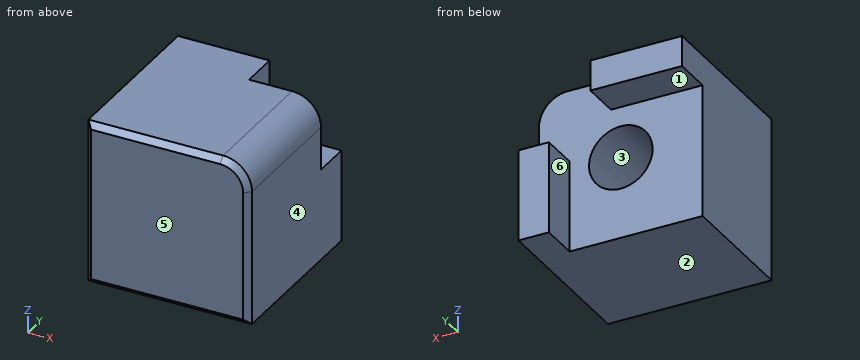
```python
from build123d import *

# Parameters (mm, degrees)
BASE_W                = 8.5
BASE_H                = 8.5
BOSS_EXTRUDE1_DEPTH   = 8.5
CUTOUT_W              = 7
CUTOUT_H              = 7
CUT_EXTRUDE1_DEPTH    = 1.5
SKETCH3_W             = 1.5
SKETCH3_H             = 1.5
CUT_EXTRUDE2_DEPTH    = 12.803071634
FILLET3_R             = 0.508
FILLET4_R             = 1.5
M4_TAPPED_HOLE1_D     = 3.3
M4_TAPPED_HOLE1_DEPTH = 5
M4_TAPPED_HOLE1_TIP   = 0.991420021
CUT_EXTRUDE3_START    = -1.5
CUT_EXTRUDE3_DEPTH    = 1.5
CHAMFER1_SIZE         = 0.3
SKETCH15_W            = 1.5875
SKETCH15_H            = 4.7625
SKETCH15_W_2          = 4.7625
SKETCH15_H_2          = 1.5875
BOSS_EXTRUDE2_DEPTH   = 2


with BuildPart() as part:
    # Base → Boss-Extrude1 (new body)
    with BuildSketch(Plane(origin=(0, 0, 0), x_dir=(1, 0, 0), z_dir=(0, 1, 0))):
        Rectangle(BASE_W, BASE_H)
    extrude(amount=-BOSS_EXTRUDE1_DEPTH)

    # Cutout → Cut-Extrude1 (cut)
    with BuildSketch(Plane(origin=(0, 0, 0), x_dir=(1, 0, 0), z_dir=(0, 1, 0))):
        with Locations((-0.75, 0.75)):
            Rectangle(CUTOUT_W, CUTOUT_H)
    extrude(amount=-CUT_EXTRUDE1_DEPTH, mode=Mode.SUBTRACT)

    # Sketch3 → Cut-Extrude2 (cut, through all)
    with BuildSketch(Plane.ZY.offset(-2.75)):
        with Locations((-3.5, -0.75)):
            Rectangle(SKETCH3_W, SKETCH3_H)
    cut_extrude2 = extrude(amount=-CUT_EXTRUDE2_DEPTH, mode=Mode.SUBTRACT)

    # Mirror1: Cut-Extrude2 across plane
    add(cut_extrude2.mirror(Plane(origin=(0, 0, 0), x_dir=(0.7071067811865476, 0, 0.7071067811865475), z_dir=(0.7071067811865475, 0, -0.7071067811865476))), mode=Mode.SUBTRACT)

    # Fillet3
    fillet3_edges = [part.edges().sort_by_distance(p)[0] for p in [
        (2.75, -0.75, 2.75),
    ]]
    fillet(fillet3_edges, radius=FILLET3_R)

    # Fillet4
    fillet4_edges = [part.edges().sort_by_distance(p)[0] for p in [
        (4.25, -4.25, 4.25),
    ]]
    fillet(fillet4_edges, radius=FILLET4_R)

    # M4 Tapped Hole1
    with Locations(Plane(origin=(0, -1.5, 0), x_dir=(1, 0, 0), z_dir=(0, 1, 0))):
        with Locations((0, 0)):
            Hole(M4_TAPPED_HOLE1_D / 2, depth=M4_TAPPED_HOLE1_DEPTH)
            with Locations((0, 0, -(M4_TAPPED_HOLE1_DEPTH + M4_TAPPED_HOLE1_TIP / 2))):  # 118° drill point
                Cone(0, M4_TAPPED_HOLE1_D / 2, M4_TAPPED_HOLE1_TIP, mode=Mode.SUBTRACT)

    # Sketch14 → Cut-Extrude3 (cut)
    with BuildSketch(Plane(origin=(0, 0, 0), x_dir=(1, 0, 0), z_dir=(0, 1, 0)).offset(CUT_EXTRUDE3_START)):
        with BuildLine():
            Line((-2.75, -4.25), (2.75, -4.25))
            ThreePointArc((2.75, -4.25), (3.810660172, -3.810660172), (4.25, -2.75))
            Line((4.25, -2.75), (4.25, 2.75))
            Line((4.25, 2.75), (2.75, 2.75))
            Line((2.75, 2.75), (2.75, -2.242))
            ThreePointArc((2.75, -2.242), (2.601210245, -2.601210245), (2.242, -2.75))
            Line((2.242, -2.75), (-2.75, -2.75))
            Line((-2.75, -2.75), (-2.75, -4.25))
        make_face()
    extrude(amount=CUT_EXTRUDE3_DEPTH, mode=Mode.SUBTRACT)

    # Chamfer1
    chamfer1_edges = [part.edges().sort_by_distance(p)[0] for p in [
        (-4.25, -8.5, 0),
        (-0.75, -8.5, 4.25),
        (4.25, -8.5, -0.75),
        (3.810660172, -8.5, 3.810660172),
        (0, -8.5, -4.25),
    ]]
    chamfer(chamfer1_edges, length=CHAMFER1_SIZE)

    # Sketch15 → Boss-Extrude2 (add)
    with BuildSketch(Plane(origin=(0, -1.5, 0), x_dir=(1, 0, 0), z_dir=(0, 1, 0))):
        with Locations((3.45625, 1.86875)):
            Rectangle(SKETCH15_W, SKETCH15_H)
        with Locations((-1.86875, -3.45625)):
            Rectangle(SKETCH15_W_2, SKETCH15_H_2)
    extrude(amount=BOSS_EXTRUDE2_DEPTH)


solid = part.part
```
The model under review builds one solid part; all positions refer to its coordinate system, in mm. Face numbers are marked on the shaded views. A direction names the side the tool comes from. Give positions to 0.01 mm unless a question says otherwise; leave off trailing zeros. Write each loop counter-clockwise with the first axis right and the second up, starting at its lowest first coordinate (ties: lowest second). Pieces come first, ordered by that corner, then holes.
(1) Consider section C-C, the plane x = -2. Give the boundary of the cut face in (y, z).
(2) To check wall thickness, follow L1, parallel to Z at x = 0, y = -5.2; L2, parallel to Y at x = -2.5, z = -3.25; L3, parallel to Z at x = -1, y = -5.5. State the ranges of each line that lie inside material, in increasing order.
(3) Tool access review of the marked faces 1 and 2: name each direction out of +Z, -Z, +X, -X, +Y, -Y from which nothing blocks a thin tool from reaching the whole face with its end or side.
(4) For P1, Ø0.5, axis at x = 3, y = 0, coming from the +Z side; P2, Ø0.8, axis at y = 0, z = 4, coming from the +X side; P3, Ø1.5, axis at x = 1, z = -2.5, coming from the +Y side, all flat-tipped, find the tip position at first contact; note any pin that passes through.
(5) Consider section A-A, the plane y = -1. Give the boundary of the cut face in (x, z).
(6) Consider section B-B, the plane y = -3.75. Give the boundary of the cut face in (x, z).
(7) The part is to be moulded in two halves that separate along X. For the marked faces 3, 4, 5 and 6, say which applies: released by +X, released by -X, zero draft, split by the parting line, or undercut.
Returned:
1. outline: (-8.5, -3.95) - (-8.2, -4.25) - (-1.5, -4.25) - (-1.5, 2.66) - (0.5, 2.66) - (0.5, 4.25) - (-8.2, 4.25) - (-8.5, 3.95) - close
2. L1: z = -4.25 to -1.65, 1.65 to 4.25
2. L2: y = -8.5 to -1.5
2. L3: z = -4.25 to -1.31, 1.31 to 4.25
3. face 1: -Z, +X, -X, +Y
3. face 2: -Z, +X, -X, +Y, -Y
4. P1: stops at z = 0.51
4. P2: stops at x = 0.51
4. P3: stops at y = -1.5
5. outline: (-4.25, 2.66) - (0.51, 2.66) - (0.51, 4.25) - (-4.25, 4.25) - close; (2.66, -4.25) - (4.25, -4.25) - (4.25, 0.51) - (2.66, 0.51) - close
6. outline: (-4.25, -4.25) - (4.25, -4.25) - (4.25, 2.75) arc R1.5 ccw to (2.75, 4.25) - (-4.25, 4.25) - close; hole circle Ø3.3 at (0, 0)
7. face 3: undercut
7. face 4: released by +X
7. face 5: zero draft
7. face 6: released by -X
